Could you check a few things on this model? Use its own coordinates, in mm. Round coordinates to 2 decimals unless told otherwise and drop trailing zeros. Loops run counter-clockwise (first coordinate to the right, second up) from the corner with the lowest first, then second, coordinate; pieces in that order, holes last. Notation, with made-up numbers: (-1.5, -25.75) -> (11.5, -25.75) arc R26 ccw to (11.5, 9.25) -> close; hole circle Ø5 at (-8, 29.25). An arc over 180 degrees is marked (long way). Write each question's results on one line, items separated by ' | '. Start each with the question number.
1) If I drill on probe 1 along Z at (x, y) = (-1, 3.75); probe 2 along X at (y, z) = (1.25, 12.25); probe 3 along Z at (x, y) = (2.25, -1.75), over which ranges is the centre line in solid material (lowest first)?
2) For P1, Ø5, axis at x = -2, z = 10.5, coming from the +Y side; P2, Ø1, axis at y = -1.5, z = 13, coming from the +X side; P3, Ø1, axis at x = 3, z = 16.5, coming from the -Y side, each with a flat end and sliding along its axis, tell me the tip position at first contact or that it passes through.
3) We'd pull the mould along Z, two halves only. Please class faces 1 (the cylindrical face through (-3, 0, 13)), 2 (the flat face through (4, 0, 4)), 3 (the conical face through (2.603, -4.483, 0.106)): pulls with the +Z half, pulls with the -Z half, needs draft (parallel to the pull), parting line crosses it, or undercut.
4) Imagine slicing it at A-A, the plane z = 5. List the corners of the cut face in (x, y) for me, plus the area to 3 significant figures.
from build123d import *

# Parameters (mm, degrees)
EXTRUDE_1_DEPTH = 4
SKETCH_2_R      = 3
EXTRUDE_2_DEPTH = 18
CHAMFER_1_SIZE  = 0.5545
FILLET_1_R      = 0.5


with BuildPart() as part:
    # Эскиз1 → Бобышка-Вытянуть1 (new body)
    with BuildSketch(Plane.XY):
        Polygon((-2.886751346, 5), (-5.773502692, 0), (-2.886751346, -5), (2.886751346, -5), (5.773502692, 0), (2.886751346, 5), align=None)
    extrude(amount=EXTRUDE_1_DEPTH)

    # Эскиз2 → Бобышка-Вытянуть2 (add)
    with BuildSketch(Plane.XY.offset(4)):
        Circle(SKETCH_2_R)
    extrude(amount=EXTRUDE_2_DEPTH)

    # Эскиз3 → Вырез-Повернуть1 (revolve, cut)
    with BuildSketch(Plane(origin=(0, 0, 0), x_dir=(0, 0, -1), z_dir=(1, 0, 0))):
        Polygon((0, 5), (0, 6.24), (-0.715914334, 6.24), align=None)
    revolve(axis=Axis((0, 0, 1000), (0, 0, -1)), mode=Mode.SUBTRACT)

    # Фаска1
    chamfer_1_edges = [part.edges().sort_by_distance(p)[0] for p in [
        (-3, 0, 22),
    ]]
    chamfer(chamfer_1_edges, length=CHAMFER_1_SIZE)

    # Скругление1
    fillet_1_edges = [part.edges().sort_by_distance(p)[0] for p in [
        (-3, 0, 4),
    ]]
    fillet(fillet_1_edges, radius=FILLET_1_R)


solid = part.part
Checked values:
1) probe 1: 0 to 4 | probe 2: -2.73 to 2.73 | probe 3: 0 to 21.6
2) P1: y = 3 | P2: x = 2.83 | P3: y = -1.66
3) face 1: needs draft | face 2: pulls with the +Z half | face 3: pulls with the -Z half
4) outline: circle Ø6 at (0, 0) | area: 28.3 mm^2
